from build123d import *

# Parameters (mm, degrees)
SKETCH1_W           = 80
SKETCH1_H           = 21
BOSS_EXTRUDE1_DEPTH = 2
BOSS_EXTRUDE2_DEPTH = 8
SKETCH3_R           = 1.6
CUT_EXTRUDE1_DEPTH  = 59.625759514
CUT_EXTRUDE2_START  = 32.087294298
SKETCH3_5_R         = 3.1
SKETCH3_5_R_2       = 1.6
CUT_EXTRUDE2_DEPTH  = 32.087294298
SKETCH4_W           = 64
SKETCH4_H           = 6
BOSS_EXTRUDE5_DEPTH = 17


with BuildPart() as part:
    # Sketch1 → Boss-Extrude1 (new body)
    with BuildSketch(Plane(origin=(0, 12.25, 0), x_dir=(1, 0, 0), z_dir=(0, 1, 0))):
        with Locations((5.518936126, -23.587294298)):
            Rectangle(SKETCH1_W, SKETCH1_H)
        Polygon((-23.081063874, -28.087294298), (34.118936126, -28.087294298), (34.118936126, -19.087294298), (7.681087054, -19.087294298), (7.681087054, -16.087294298), (3.181087054, -16.087294298), (3.181087054, -19.087294298), (-23.081063874, -19.087294298), align=None, mode=Mode.SUBTRACT)
    extrude(amount=BOSS_EXTRUDE1_DEPTH)

    # Sketch2 → Boss-Extrude2 (add)
    with BuildSketch(Plane.ZY.offset(34.481063874)):
        Polygon((34.087294298, 12.25), (34.087294298, -4.75), (28.087294298, -4.75), (13.087294298, 12.25), align=None)
    boss_extrude2 = extrude(amount=-BOSS_EXTRUDE2_DEPTH)

    # Sketch3 → Cut-Extrude1 (cut, symmetric)
    with BuildSketch(Plane.XY):
        with Locations(Location((-30.481063874, 5.25, 0), (0, 0, 90))):
            Circle(SKETCH3_R)
    cut_extrude1 = extrude(amount=CUT_EXTRUDE1_DEPTH, both=True, mode=Mode.SUBTRACT)

    # Sketch3<5> → Cut-Extrude2 (cut)
    with BuildSketch(Plane.XY.offset(CUT_EXTRUDE2_START)):
        with Locations(Location((-30.481063874, 5.25, 0), (0, 0, 180))):
            Circle(SKETCH3_5_R)
        with Locations(Location((-30.481063874, 5.25, 0), (0, 0, 180))):
            Circle(SKETCH3_5_R_2, mode=Mode.SUBTRACT)
    cut_extrude2 = extrude(amount=-CUT_EXTRUDE2_DEPTH, mode=Mode.SUBTRACT)

    # Mirror1: Boss-Extrude2, Cut-Extrude1, Cut-Extrude2 across plane
    add(boss_extrude2.mirror(Plane.ZY.offset(-5.518936126)))
    add(cut_extrude1.mirror(Plane.ZY.offset(-5.518936126)), mode=Mode.SUBTRACT)
    add(cut_extrude2.mirror(Plane.ZY.offset(-5.518936126)), mode=Mode.SUBTRACT)

    # Sketch4 → Boss-Extrude5 (add)
    with BuildSketch(Plane.XZ.offset(-12.25)):
        with Locations((5.518936126, 31.087294298)):
            Rectangle(SKETCH4_W, SKETCH4_H)
    extrude(amount=BOSS_EXTRUDE5_DEPTH)


solid = part.part
Part model, mm, in its own coordinate system. A direction names the side the tool comes from. Round coordinates to 2 decimals unless told otherwise and drop trailing zeros. Write each loop counter-clockwise with the first axis right and the second up, starting at its lowest first coordinate (ties: lowest second). Pieces come first, ordered by that corner, then holes. Notation, with made-up numbers: (62.25, 50.5) - (89.25, 50.5) arc R15 cw to (89.25, 63.5) - close; hole circle Ø3 at (59.25, -27). An arc over 180 degrees is marked (long way). Use CSV: the item, a comma, the result in double quotes.
Item 1: Slice it at B-B, the plane z = 22.5. Write the cut outline in (x, y), then the cut area to 3 significant figures.
Results list:
outline,"(-34.48, 1.58) - (-26.48, 1.58) - (-26.48, 12.25) - (-23.08, 12.25) - (-23.08, 14.25) - (-34.48, 14.25) - close; (34.12, 12.25) - (37.52, 12.25) - (37.52, 1.58) - (45.52, 1.58) - (45.52, 14.25) - (34.12, 14.25) - close; hole circle Ø6.2 at (-30.48, 5.25); hole circle Ø6.2 at (41.52, 5.25)"
area,"156 mm²"
Item 2: Slice it at A-A, the plane x = 11. Write the cut outline in (y, z).
Results list:
outline,"(-4.75, 28.09) - (14.25, 28.09) - (14.25, 34.09) - (-4.75, 34.09) - close; (12.25, 13.09) - (14.25, 13.09) - (14.25, 19.09) - (12.25, 19.09) - close"
Item 3: Tool access for faces 5 (the flat face through (-26.481, 6, 22)), 6 (the flat face through (43, 7, 32.087)), 7 (the flat face through (-10, 13, 19.087)), 8 (the flat face through (5, 14.25, 30)): list every direction of +Z, -Z, +X, -X, +Y, -Y with a clear straight run to the whole face (end or side of a thin tool).
Results list:
face 5,"-Z, -Y"
face 6,"-Z"
face 7,"+Y, -Y"
face 8,"+Z, -Z, +X, -X, +Y"
Item 4: Flat gauge pins, fed straight in: P1, Ø1, axis at x = 7, y = 5.5, coming from the -Z side; P2, Ø3.5, axis at x = -30.48, y = 5.25, coming from the -Z side; P3, Ø10, axis at x = 26, z = 20.5, coming from the -Y side. Where does each tip first touch, or does it go through?
Results list:
P1,"stops at z = 28.09"
P2,"stops at z = 32.09"
P3,"stops at y = 12.25"
Item 5: Slice it at D-D, the plane y = 5.25. Write the cut outline in (x, z).
Results list:
outline,"(-34.48, 19.26) - (-33.58, 19.26) - (-33.58, 32.09) - (-32.08, 32.09) - (-32.08, 34.09) - (-34.48, 34.09) - close; (-28.88, 32.09) - (-27.38, 32.09) - (-27.38, 19.26) - (-26.48, 19.26) - (-26.48, 28.09) - (37.52, 28.09) - (37.52, 19.26) - (38.42, 19.26) - (38.42, 32.09) - (39.92, 32.09) - (39.92, 34.09) - (-28.88, 34.09) - close; (43.12, 32.09) - (44.62, 32.09) - (44.62, 19.26) - (45.52, 19.26) - (45.52, 34.09) - (43.12, 34.09) - close"
Item 6: Pull direction Z, two halves, no side cores. Call faces 1 (the flat face through (5, 5, 34.087)), 2 (the flat face through (34.119, 13, 24)), 3 (the flat face through (5, 13, 13.087)), 4 (the flat face through (5, 13, 16.087)): pulls with the +Z half, pulls with the -Z half, needs draft (parallel to the pull), parting line crosses it, or undercut.
Results list:
face 1,"pulls with the +Z half"
face 2,"undercut"
face 3,"pulls with the -Z half"
face 4,"undercut"
Item 7: Slice it at C-C, the plane z = 30.5. Write the cut outline in (x, y), then the cut area to 3 significant figures.
Results list:
outline,"(-34.48, -4.75) - (45.52, -4.75) - (45.52, 14.25) - (-34.48, 14.25) - close; hole circle Ø6.2 at (-30.48, 5.25); hole circle Ø6.2 at (41.52, 5.25)"
area,"1,460 mm²"
Item 8: Wall check: L1, parallel to X at y = 5.25, z = 21.5; L2, parallel to X at y = 5.25, z = 33.1; L3, parallel to X at y = 9.25, z = 20. Give the ranges that are in metal, low to high.
Results list:
L1,"x = -34.48 to -33.58, -27.38 to -26.48, 37.52 to 38.42, 44.62 to 45.52"
L2,"x = -34.48 to -32.08, -28.88 to 39.92, 43.12 to 45.52"
L3,"x = -34.48 to -26.48, 37.52 to 45.52"
